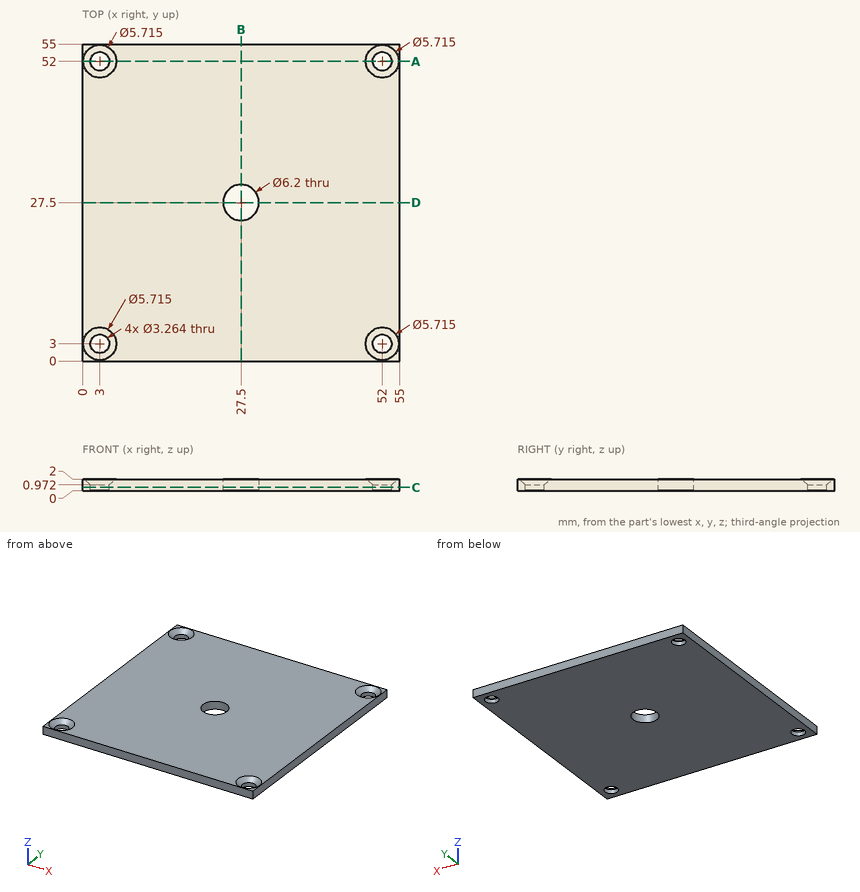
Here's the drawing with two shaded views (mm, measured from the low corner). I have some questions. Round coordinates to 2 decimals unless told otherwise and drop trailing zeros. Loops run counter-clockwise (first coordinate to the right, second up) from the corner with the lowest first, then second, coordinate; pieces in that order, holes last.
Item 1: Suppose I cut it at A-A, the plane y = 52. Write out the boundary of the cut face in (x, z).
Item 2: Suppose I cut it at B-B, the plane x = 27.5. Write out the boundary of the cut face in (y, z).
Item 3: Suppose I cut it at C-C, the plane z = 0.55. Write out the boundary of the cut face in (x, y).
Item 4: Please list where these lines run through material, in increasing order: L1, parallel to X at y = 52, z = 0.75; L2, parallel to X at y = 50, z = 1.7.
Reported:
1. outline: (0, 0) - (1.37, 0) - (1.37, 0.97) - (0.14, 2) - (0, 2) - close; (4.63, 0) - (50.37, 0) - (50.37, 0.97) - (49.14, 2) - (5.86, 2) - (4.63, 0.97) - close; (53.63, 0) - (55, 0) - (55, 2) - (54.86, 2) - (53.63, 0.97) - close
2. outline: (0, 0) - (24.4, 0) - (24.4, 2) - (0, 2) - close; (30.6, 0) - (55, 0) - (55, 2) - (30.6, 2) - close
3. outline: (0, 0) - (55, 0) - (55, 55) - (0, 55) - close; hole circle Ø3.26 at (3, 3); hole circle Ø3.26 at (3, 52); hole circle Ø6.2 at (27.5, 27.5); hole circle Ø3.26 at (52, 3); hole circle Ø3.26 at (52, 52)
4. L1: x = 0 to 1.37, 4.63 to 50.37, 53.63 to 55
4. L2: x = 0 to 1.5, 4.5 to 50.5, 53.5 to 55
